Verification items for this drawing (mm, ordinates from the low corner). Coordinates: 2 decimals unless noted, no trailing zeros. Loops run counter-clockwise (first coordinate to the right, second up) from the corner with the lowest first, then second, coordinate; pieces in that order, holes last. Notation, with made-up numbers: M 19,70 L 38,70 A11 ccw 38,89 Z; hole C 34,70 d1. An arc over 180 degrees is marked long. Return JSON: item names as keys, results as strings.
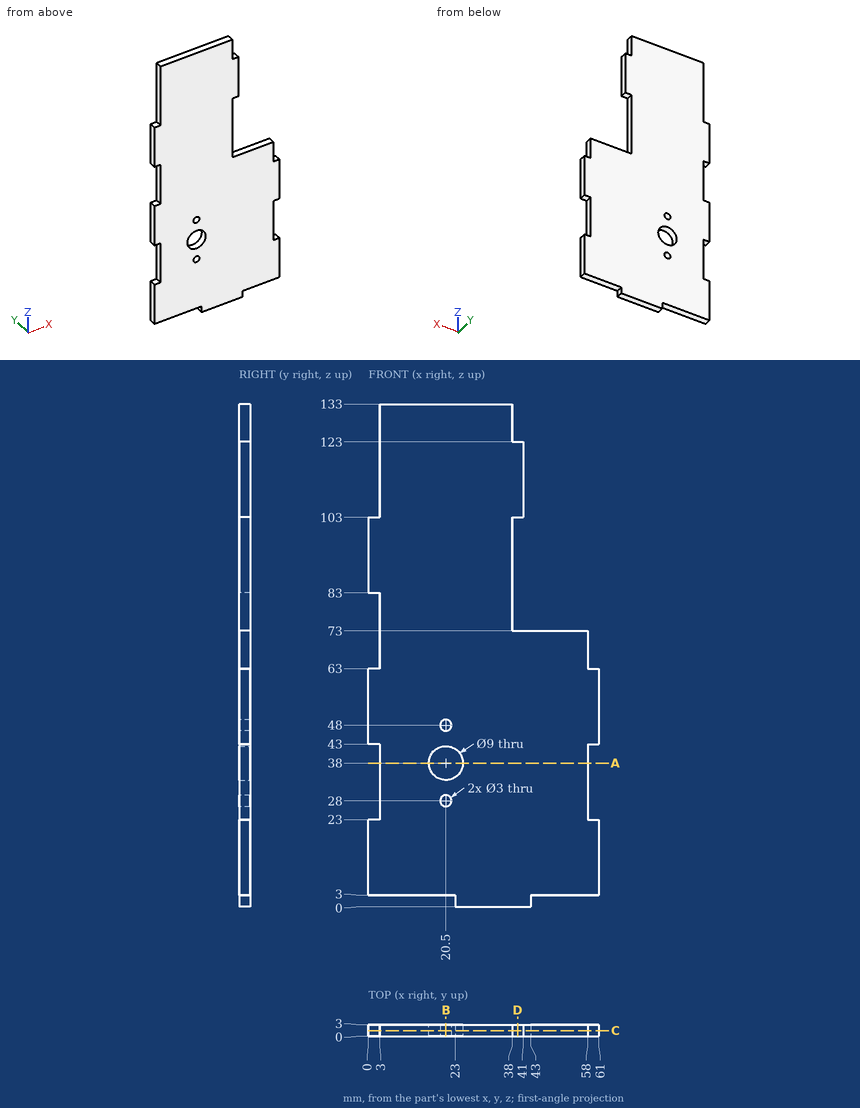
1) Section check C-C on y = 1.4. Count the separate pieces of the cut face and the enclosed holes in it, then the cut area to 3 significant figures.
Answers:
{"separate pieces": "1", "enclosed holes": "3", "area": "6,290 mm²"}
2) Section check B-B on x = 20.5. Record the cut outline in (y, z), then the cut area to 3 significant figures.
Answers:
{"outline": "M 0,3 L 3,3 L 3,26.5 L 0,26.5 Z; M 0,29.5 L 3,29.5 L 3,33.5 L 0,33.5 Z; M 0,42.5 L 3,42.5 L 3,46.5 L 0,46.5 Z; M 0,49.5 L 3,49.5 L 3,133 L 0,133 Z", "area": "345 mm²"}
3) Section check D-D on x = 39.5. Record the cut outline in (y, z), then the cut area to 3 significant figures.
Answers:
{"outline": "M 0,0 L 3,0 L 3,73 L 0,73 Z; M 0,103 L 3,103 L 3,123 L 0,123 Z", "area": "279 mm²"}
4) Scan lines: line 1 along Z through (x, y) = (39.5, 1); line 2 along X through (y, z) = (1.4, 28); line 3 along Z through (x, y) = (10, 1.5). Record each from-to range of solid material in increasing order. Write a range as [from, to].
Answers:
{"line 1": "[0, 73], [103, 123]", "line 2": "[3, 19], [22, 58]", "line 3": "[3, 133]"}
5) Section check A-A on z = 38. Record the cut outline in (x, y).
Answers:
{"outline": "M 3,0 L 16,0 L 16,3 L 3,3 Z; M 25,0 L 58,0 L 58,3 L 25,3 Z"}
6) Go/stop test with flat-tipped pins: pin 1 Ø0.9 at (x, y) = (1.5, 1) entering from -Z; pin 2 Ø0.9 at (x, y) = (47, 1.5) entering from +Z; pin 3 Ø0.9 at (y, z) = (2, 37.5) entering from +X. Record where each tip stops, or that it passes through.
Answers:
{"pin 1": "z = 3", "pin 2": "z = 73", "pin 3": "x = 58"}
